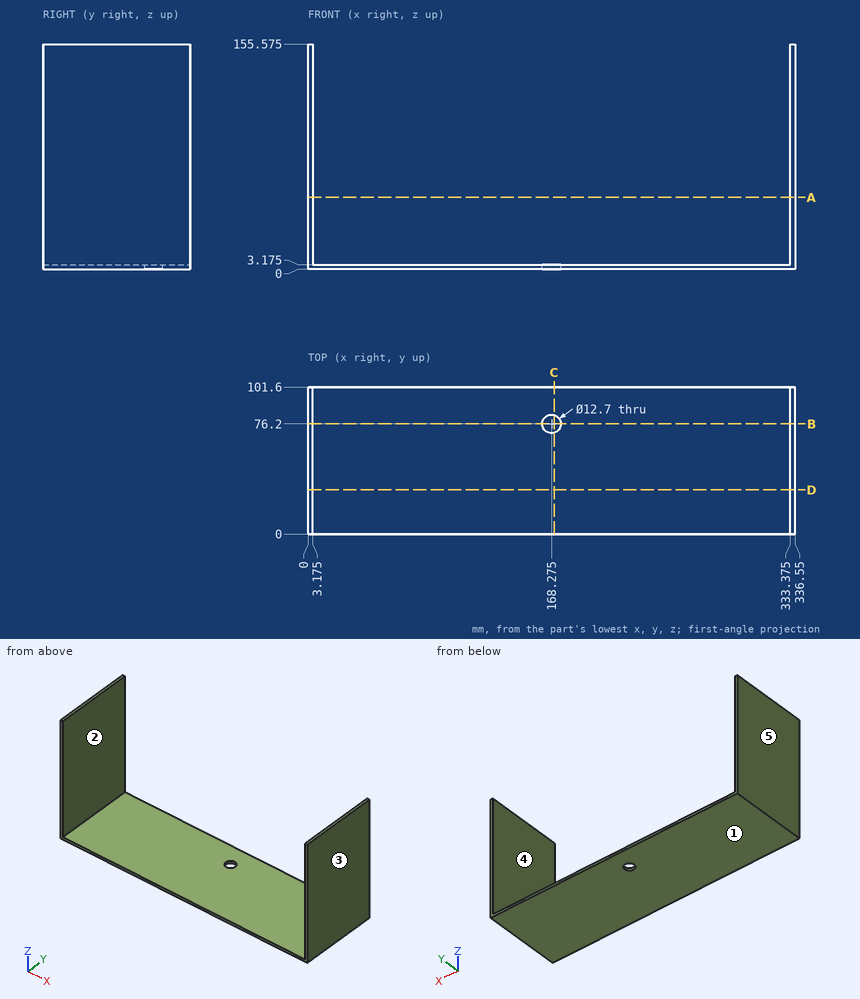
The drawing under review shows one solid part. Ordinate dimensions are in mm from its lowest x, y, z. A direction names the side the tool comes from. Round coordinates to 2 decimals unless told otherwise and drop trailing zeros. Order: outer loops, then holes, each group sorted by start corner. A loop starts at its lowest first (then second) coordinate and runs counter-clockwise, first axis right, second up. Notation, with made-up numbers: (-5.75, -23.5) -> (34.25, -23.5) arc R27 ccw to (34.25, 10.5) -> close; hole circle Ø5 at (26, 32.25). An arc over 180 degrees is marked (long way). Return JSON: item names as keys, results as strings.
1. The part is to be moulded in two halves that separate along X. For the marked faces 1, 2 and 3, say which applies: +X half, -X half, draft (parallel to the pull), parting line (faces both ways), or undercut.
Answer block:
{"face 1": "draft", "face 2": "undercut", "face 3": "+X half"}
2. For the marked faces 4 and 5, list the 3-axis set-ups (+Z, -Z, +X, -X, +Y, -Y) from which the entire face can be reached by the end or side of a thin tool; tool diameter is ignored.
Answer block:
{"face 4": "+Z, +Y, -Y", "face 5": "+Z, -Z, -X, +Y, -Y"}
3. Take a section at B-B (y = 76.2). Write out the cut boundary in (x, z) (3 decimals), then the cut area to 3 significant figures.
Answer block:
{"outline": "(0, 0) -> (161.925, 0) -> (161.925, 3.175) -> (3.175, 3.175) -> (3.175, 155.575) -> (0, 155.575) -> close; (174.625, 0) -> (336.55, 0) -> (336.55, 155.575) -> (333.375, 155.575) -> (333.375, 3.175) -> (174.625, 3.175) -> close", "area": "2,000 mm²"}
4. Take a section at C-C (x = 170). Write out the cut boundary in (y, z) (3 decimals).
Answer block:
{"outline": "(0, 0) -> (70.089, 0) -> (70.089, 3.175) -> (0, 3.175) -> close; (82.311, 0) -> (101.6, 0) -> (101.6, 3.175) -> (82.311, 3.175) -> close"}
5. Insertion check: P1, Ø5, axis at x = 207, y = 40.5, coming from the +Z side (3 decimals). The pin has a flat end and moves straight along its axis. Give the tip position at first contact, or say it passes through.
Answer block:
{"P1": "stops at z = 3.175"}
6. For L1, parallel to X at y = 15, z = 10 (3 decimals); L2, parallel to X at y = 76, z = 1; L3, parallel to Z at x = 294.5, y = 48.5 (3 decimals), list the stretches that pass through material, from the lowest coordinate up. Write a range as [from, to].
Answer block:
{"L1": "x = [0, 3.175], [333.375, 336.55]", "L2": "x = [0, 161.93], [174.62, 336.55]", "L3": "z = [0, 3.175]"}
7. Take a section at A-A (z = 49.5). Write out the cut boundary in (x, y) (3 decimals).
Answer block:
{"outline": "(0, 0) -> (3.175, 0) -> (3.175, 101.6) -> (0, 101.6) -> close; (333.375, 0) -> (336.55, 0) -> (336.55, 101.6) -> (333.375, 101.6) -> close"}
8. Take a section at D-D (y = 30.5). Write out the cut boundary in (x, z) (3 decimals).
Answer block:
{"outline": "(0, 0) -> (336.55, 0) -> (336.55, 155.575) -> (333.375, 155.575) -> (333.375, 3.175) -> (3.175, 3.175) -> (3.175, 155.575) -> (0, 155.575) -> close"}
